```python
from build123d import *

# Parameters (mm, degrees)
SKETCH1_R           = 28.5
SKETCH1_R_2         = 21
BOSS_EXTRUDE1_DEPTH = 60.675
SKETCH2_R           = 2.25
CUT_EXTRUDE1_DEPTH  = 73.841990809
CIRPATTERN1_COUNT   = 4
CUT_EXTRUDE4_START  = -1
SKETCH5_R           = 28.5
CUT_EXTRUDE4_DEPTH  = 1
SKETCH3_R           = 2.25
CUT_EXTRUDE2_DEPTH  = 6.5
SKETCH4_R           = 24.5
CUT_EXTRUDE3_DEPTH  = 109.85


with BuildPart() as part:
    # Sketch1 → Boss-Extrude1 (new, symmetric)
    with BuildSketch(Plane(origin=(0, 0, 0), x_dir=(1, 0, 0), z_dir=(0, 1, 0))):
        with Locations(Location((0, 0, 0), (0, 0, 270))):
            Circle(SKETCH1_R)
        with Locations(Location((0, 0, 0), (0, 0, 270))):
            Circle(SKETCH1_R_2, mode=Mode.SUBTRACT)
    extrude(amount=BOSS_EXTRUDE1_DEPTH, both=True)

    # Sketch2 → Cut-Extrude1 (cut, through all)
    with BuildSketch(Plane.XY):
        with Locations(Location((0, 55.675, 0), (0, 0, 90))):
            Circle(SKETCH2_R)
    cut_extrude1 = extrude(amount=-CUT_EXTRUDE1_DEPTH, mode=Mode.SUBTRACT)

    # CirPattern1: Cut-Extrude1 ×4 about axis
    cirpattern1_axis = Axis((0, 60.675, 0), (0, -1, 0))
    for i in range(1, CIRPATTERN1_COUNT):
        add(cut_extrude1.rotate(cirpattern1_axis, i * 360 / CIRPATTERN1_COUNT), mode=Mode.SUBTRACT)

    # Sketch5 → Cut-Extrude4 (cut)
    with BuildSketch(Plane.XZ.offset(60.675).offset(CUT_EXTRUDE4_START)):
        with Locations(Location((0, 0, 0), (0, 0, 270))):
            Circle(SKETCH5_R)
    extrude(amount=CUT_EXTRUDE4_DEPTH, mode=Mode.SUBTRACT)

    # Sketch3 → Cut-Extrude2 (cut)
    with BuildSketch(Plane.XZ.offset(59.675)):
        with Locations(Location((0, 24.75, 0), (0, 0, 270))):
            Circle(SKETCH3_R)
        with Locations(Location((24.75, 0, 0), (0, 0, 270))):
            Circle(SKETCH3_R)
        with Locations(Location((0, -24.75, 0), (0, 0, 270))):
            Circle(SKETCH3_R)
        with Locations(Location((-24.75, 0, 0), (0, 0, 270))):
            Circle(SKETCH3_R)
    extrude(amount=-CUT_EXTRUDE2_DEPTH, mode=Mode.SUBTRACT)

    # Sketch4 → Cut-Extrude3 (cut)
    with BuildSketch(Plane(origin=(0, 60.675, 0), x_dir=(1, 0, 0), z_dir=(0, 1, 0))):
        with Locations(Location((0, 0, 0), (0, 0, 270))):
            Circle(SKETCH4_R)
    extrude(amount=-CUT_EXTRUDE3_DEPTH, mode=Mode.SUBTRACT)


solid = part.part
```
Build history of the part. All positions in model axes, mm. A direction names the side the tool comes from. Round coordinates to 2 decimals unless told otherwise and drop trailing zeros. Order: outer loops, then holes, each group sorted by start corner. A loop starts at its lowest first (then second) coordinate and runs counter-clockwise, first axis right, second up. Notation, with made-up numbers: (35, -13.5) -> (42, -13.5) arc R16 cw to (42, 8.5) -> close; hole circle Ø7 at (-4.5, 45.25). An arc over 180 degrees is marked (long way). Answer in a Markdown table with one row per item.
1) Which spindle directions (+Z, -Z, +X, -X, +Y, -Y) get a long thin tool onto all of the face, cutting with end or side? Do faces 1 (the cylindrical face through (0.676, -56.47, 22.604)), 2 (the cylindrical face through (7.36, 6.52, 23.37)), 3 (the cylindrical face through (-0.862, 57.753, 26.42)). Say none if no direction does.
Values:
| item | result |
|---|---|
| face 1 | -Y |
| face 2 | +Y |
| face 3 | +Z, -Z |
2) Band-saw the part on D-D on z = 13.5. Give the cut face in (x, y) (3 decimals).
Values:
| item | result |
|---|---|
| outline | (-25.1, -59.675) -> (-16.086, -59.675) -> (-16.086, -49.175) -> (-20.445, -49.175) -> (-20.445, 60.675) -> (-25.1, 60.675) -> close; (16.086, -59.675) -> (25.1, -59.675) -> (25.1, 60.675) -> (20.445, 60.675) -> (20.445, -49.175) -> (16.086, -49.175) -> close |
3) Band-saw the part on A-A on x = 0. Give the cut face in (y, z) (3 decimals), and give its area (3 significant figures).
Values:
| item | result |
|---|---|
| outline | (-59.675, -28.5) -> (53.425, -28.5) -> (53.425, -24.5) -> (-49.175, -24.5) -> (-49.175, -21) -> (-59.675, -21) -> (-59.675, -22.5) -> (-53.175, -22.5) -> (-53.175, -27) -> (-59.675, -27) -> close; (-59.675, 21) -> (-49.175, 21) -> (-49.175, 24.5) -> (53.425, 24.5) -> (53.425, 28.5) -> (-59.675, 28.5) -> (-59.675, 27) -> (-53.175, 27) -> (-53.175, 22.5) -> (-59.675, 22.5) -> close; (57.925, -28.5) -> (60.675, -28.5) -> (60.675, -24.5) -> (57.925, -24.5) -> close; (57.925, 24.5) -> (60.675, 24.5) -> (60.675, 28.5) -> (57.925, 28.5) -> close |
| area | 942 mm2 |
4) Wall check: L1, parallel to X at y = -56.5, z = 0; L2, parallel to Z at x = 0, y = 27; L3, parallel to X at y = -28.5, z = 1. Give the ranges that are in metal, low to high.
Values:
| item | result |
|---|---|
| L1 | -28.5 to -27, -22.5 to -21, 21 to 22.5, 27 to 28.5 |
| L2 | -28.5 to -24.5, 24.5 to 28.5 |
| L3 | -28.48 to -24.48, 24.48 to 28.48 |
5) Mould opens along Y. For faces 4 (the cylindrical face through (22.554, -56.47, 0.488)), 5 (the flat face through (0, -53.175, -25)), 6 (the cylindrical face through (0.862, 57.753, -26.42)) say: released by +Y, released by -Y, zero draft, split by the parting line, or undercut.
Values:
| item | result |
|---|---|
| face 4 | zero draft |
| face 5 | released by -Y |
| face 6 | undercut |
6) Pin check, flat tips, straight feed: P1, Ø1.5, axis at y = -15.5, z = 14, coming from the -X side; P2, Ø4, axis at y = 39.5, z = 20.5, coming from the -X side; P3, Ø7, axis at y = 55.675, z = 0, coming from the -X side; P4, Ø2, axis at x = 1.5, y = -9, coming from the +Z side. Stop position of each tip, or through.
Values:
| item | result |
|---|---|
| P1 | x = -25.23 |
| P2 | x = -21.68 |
| P3 | x = -28.5 |
| P4 | z = 28.5 |
7) Band-saw the part on C-C on x = -9. Give the cut face in (y, z) (3 decimals).
Values:
| item | result |
|---|---|
| outline | (-59.675, -27.042) -> (60.675, -27.042) -> (60.675, -22.787) -> (-49.175, -22.787) -> (-49.175, -18.974) -> (-59.675, -18.974) -> close; (-59.675, 18.974) -> (-49.175, 18.974) -> (-49.175, 22.787) -> (60.675, 22.787) -> (60.675, 27.042) -> (-59.675, 27.042) -> close |
8) Band-saw the part on B-B on z = 0. Give the cut face in (x, y) (3 decimals), and give its area (3 significant figures).
Values:
| item | result |
|---|---|
| outline | (-28.5, -59.675) -> (-27, -59.675) -> (-27, -53.175) -> (-22.5, -53.175) -> (-22.5, -59.675) -> (-21, -59.675) -> (-21, -49.175) -> (-24.5, -49.175) -> (-24.5, 53.425) -> (-28.5, 53.425) -> close; (-28.5, 57.925) -> (-24.5, 57.925) -> (-24.5, 60.675) -> (-28.5, 60.675) -> close; (21, -59.675) -> (22.5, -59.675) -> (22.5, -53.175) -> (27, -53.175) -> (27, -59.675) -> (28.5, -59.675) -> (28.5, 53.425) -> (24.5, 53.425) -> (24.5, -49.175) -> (21, -49.175) -> close; (24.5, 57.925) -> (28.5, 57.925) -> (28.5, 60.675) -> (24.5, 60.675) -> close |
| area | 942 mm2 |
